Autodesk Inventor part; units mm, degrees
ref_plane "YZ Plane" through (0, 0, 0) normal (1, 0, 0) x (0, 1, 0)
ref_plane "XZ Plane" through (0, 0, 0) normal (0, 1, 0) x (-1, 0, 0)
ref_plane "XY Plane" through (0, 0, 0) normal (0, 0, 1) x (1, 0, 0)
sketch "Sketch1" plane through (0, 0, 0) normal (0, 1, 0) x (-1, 0, 0)
  circle A0 centre (0, 0) radius 11
  circle A1 centre (0, 0) radius 1.5
  circle A2 centre (0, 0) radius 2
  circle A3 centre (0, 0) radius 8
  circle A4 centre (0, 0) radius 7
  circle A5 centre (0, 0) radius 9
  dimension "d0" = 22
  dimension "d5" = 3
  dimension "d8" = 4
  dimension "d14" = 16
  dimension "d15" = 14
  dimension "d16" = 18
extrude "Extrusion1" add sketch "Sketch1" along normal blind 13.2 contours A0 | A1 | A2 | A3 | A4 | A5
shell "Shell1" thickness 2 removed faces 1 at (3.2467, 13.2, -1.704)
fillet "Fillet1" radius 0.5 3 edges at (11, 13.2, 0) (9, 13.2, 0) (11, 0, 0)
extrude "Extrusion2" cut sketch "Sketch1" along normal through all contours A1
extrude "Extrusion3" add sketch "Sketch1" along normal blind 5 contours A0 | A3 | A4 | A5
extrude "Extrusion4" add sketch "Sketch1" along normal blind 13.2 contours A2
fillet "Fillet2" radius 1 1 edges at (11, 0, 0)
extrude "Extrusion5" cut sketch "Sketch1" along normal blind 1 contours A3
extrude "Extrusion6" cut sketch "Sketch1" along normal blind 2 contours A5
properties part number "Kolo"
Part model, mm, in its own coordinate system. A direction names the side the tool comes from. Give positions to 0.01 mm unless a question says otherwise; leave off trailing zeros. Write each loop counter-clockwise with the first axis right and the second up, starting at its lowest first coordinate (ties: lowest second). Pieces come first, ordered by that corner, then holes. Notation, with made-up numbers: M 76,1.5 L 93,1.5 A20 cw 93,32.5 Z; hole C -37.5,51 d6. An arc over 180 degrees is marked long. Use CSV: the item, a comma, the result in double quotes.
Item 1: Slice it at C-C on y = 4.5. Write the cut outline in (x, z).
Taken from the geometry:
outline,"C 0,0 d22; hole C 0,0 d3"
Item 2: Drill centre lines: probe 1 along Z at (x, y) = (0, 0.95); probe 2 along Z at (x, y) = (0, 7.75); probe 3 along X at (y, z) = (8.25, 0.25). Where is each one in solid material? Low to high.
Taken from the geometry:
probe 1,"z = -11 to -9, -7 to -1.5, 1.5 to 7, 9 to 11"
probe 2,"z = -11 to -9, -2 to -1.5, 1.5 to 2, 9 to 11"
probe 3,"x = -11 to -9, -1.98 to -1.48, 1.48 to 1.98, 9 to 11"
Item 3: Pull direction Z, two halves, no side cores. Call faces 4 (the face through (1.73, 1.49, 7.81)), 5 (the face through (9, 0, 2)), 6 (the face through (2.38, 6.77, 10.74)): +Z half, -Z half, draft (parallel to the pull), parting line (faces both ways), or undercut.
Taken from the geometry:
face 4,"undercut"
face 5,"draft"
face 6,"parting line"
Item 4: Pin check, flat tips, straight feed: P1, Ø2, axis at x = 0, z = -2.5, coming from the +Y side; P2, Ø1, axis at x = 1.5, y = 3, coming from the +Z side; P3, Ø1, axis at y = 6, z = -1, coming from the +X side; P4, Ø5, axis at x = -5, y = 8.5, coming from the -Z side. Stop position of each tip, or through.
Taken from the geometry:
P1,"stops at y = 13.2"
P2,"stops at z = 10.95"
P3,"stops at x = 10.99"
P4,"stops at z = -10.71"
Item 5: Which spindle directions (+Z, -Z, +X, -X, +Y, -Y) get a long thin tool onto all of the face, cutting with end or side? Do faces 1 (the face through (5, 13.2, -9)), 2 (the face through (-6.466, 0.493, 2.681)), 3 (the face through (1.172, 8.796, -8.923)). Say none if no direction does.
Taken from the geometry:
face 1,"+Z, -Z, +X, -X, +Y"
face 2,"-Y"
face 3,"+Y"
Item 6: Slice it at D-D on y = 6.75. Write the cut outline in (x, z).
Taken from the geometry:
outline,"C 0,0 d22; C 0,0 d4; hole C 0,0 d18; hole C 0,0 d3"
